Source: CAD feature listing. Evaluate the final solid. Frame: model axes, mm. Face numbers are marked on the shaded views. A direction names the side the tool comes from. Coordinates: 2 decimals unless noted, no trailing zeros. Loops run counter-clockwise (first coordinate to the right, second up) from the corner with the lowest first, then second, coordinate; pieces in that order, holes last. Notation, with made-up numbers: (28.5, -37) -> (76.5, -37) arc R5 ccw to (76.5, -29) -> close; hole circle Ø3 at (76, -2). An arc over 180 degrees is marked (long way). Answer as CSV lines item,"result".
from build123d import *

# Parameters (mm, degrees)
F1_DEPTH = 6.35
F3_DEPTH = 31.75
F5_DEPTH = 25.4
F6_R     = 2.5
F7_DEPTH = 25.4
F8_R     = 6.35


with BuildPart() as f1:
    # F0 (on Front) → F1 (new body)
    with BuildSketch(Plane.XZ):
        Polygon((0, 84.328), (0, 0), (26.416, 0), (33.3502, 46.99), (6.35, 71.628), (6.35, 84.328), align=None)
    extrude(amount=F1_DEPTH)

    # F2 (on face) → F3 (join)
    with BuildSketch(Plane.XZ.offset(6.35)):
        Polygon((0, 84.328), (0, 0), (6.35, 0), (6.35, 71.628), (6.35, 84.328), align=None)
    extrude(amount=F3_DEPTH)

    # F4 (on face) → F5 (cut)
    with BuildSketch(Plane.XZ.offset(6.35)):
        with BuildLine():
            Line((19.558, 12.9921), (14.478, 12.9921))
            ThreePointArc((14.478, 12.9921), (10.5029, 9.017), (14.478, 5.0419))
            Line((14.478, 5.0419), (19.558, 5.0419))
            ThreePointArc((19.558, 5.0419), (23.5331, 9.017), (19.558, 12.9921))
        make_face()
        with BuildLine():
            Line((24.1046, 45.9359), (19.0246, 45.9359))
            ThreePointArc((19.0246, 45.9359), (15.0495, 41.9608), (19.0246, 37.9857))
            Line((19.0246, 37.9857), (24.1046, 37.9857))
            ThreePointArc((24.1046, 37.9857), (28.0797, 41.9608), (24.1046, 45.9359))
        make_face()
    extrude(amount=-F5_DEPTH, mode=Mode.SUBTRACT)

    # F6 (on face) → F7 (cut)
    with BuildSketch(Plane.YZ.offset(6.35)):
        with Locations((-23.8125, 46.228)):
            Circle(F6_R)
        with Locations((-23.8125, 72.898)):
            Circle(F6_R)
    extrude(amount=-F7_DEPTH, mode=Mode.SUBTRACT)

    # F8
    f8_edges = [f1.edges().sort_by_distance(p)[0] for p in [
        (26.416, -3.175, 0),
        (33.3502, -3.175, 46.99),
        (6.35, -3.175, 71.628),
        (3.175, 0, 84.328),
        (3.175, -38.1, 84.328),
        (3.175, -38.1, 0),
    ]]
    fillet(f8_edges, radius=F8_R)


solid = f1.part
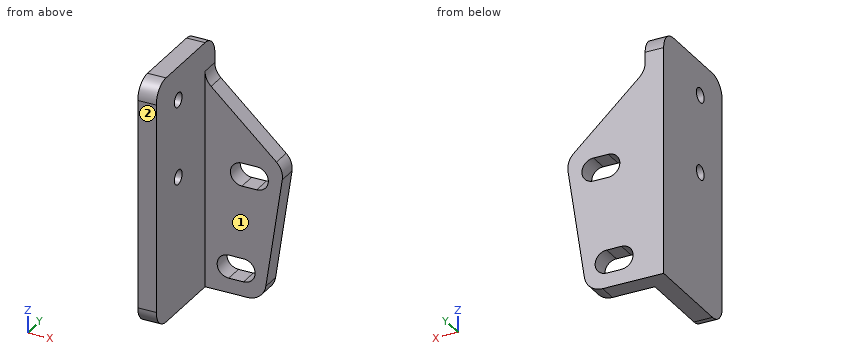
(1) Cut plane A-A (x = 22). Return the cut outline in (y, z).
Computed values:
outline,"(-6.35, 0.09) -> (0, 0.09) -> (0, 5.88) -> (-6.35, 5.88) -> close; (-6.35, 12.15) -> (0, 12.15) -> (0, 37.99) -> (-6.35, 37.99) -> close; (-6.35, 45.94) -> (0, 45.94) -> (0, 57.35) -> (-6.35, 57.35) -> close"
(2) Access query for the marked faces 1 and 2. Directions: +Z, -Z, +X, -X, +Y, -Y. A direction counts if a zero-diameter tool reaches every point of the face in a straight line with its end or side. Return the directions, or none.
Computed values:
face 1,"+Z, -Z, +X, -Y"
face 2,"+Z, -Z, +X, -X, -Y"
(3) Cut plane C-C (y = -22.5). Return the cut outline in (x, z).
Computed values:
outline,"(0, 0) -> (6.35, 0) -> (6.35, 44.1) -> (0, 44.1) -> close; (0, 48.36) -> (6.35, 48.36) -> (6.35, 70.77) -> (0, 70.77) -> close; (0, 75.03) -> (6.35, 75.03) -> (6.35, 84.33) -> (0, 84.33) -> close"
(4) Cut plane B-B (z = 11). Return the cut outline in (x, y), then the cut area to 3 significant figures.
Computed values:
outline,"(0, -38.1) -> (6.35, -38.1) -> (6.35, -6.35) -> (11.03, -6.35) -> (11.03, 0) -> (0, 0) -> close; (23, -6.35) -> (28.04, -6.35) -> (28.04, 0) -> (23, 0) -> close"
area,"304 mm^2"
(5) Material intervals for L1, parallel to Z at x = 19.5, y = -6; L2, parallel to X at y = -7.5, z = 23; L3, parallel to Y at x = 20, z = 52, sorted ascending. Write a range as [from, to].
Computed values:
L1,"[0, 5.04], [12.99, 37.99], [45.94, 59.63]"
L2,"[0, 6.35]"
L3,"[-6.35, 0]"
(6) Pin query (flat end, axial travel): pin 1 Ø8 at (y, z) = (-27.5, 33.5) entering from -X; pin 2 Ø5.5 at (x, y) = (17.5, -2.5) entering from +Z; pin 3 Ø11.5 at (y, z) = (-18.5, 48.5) entering from +X; pin 4 Ø13.5 at (x, z) = (24.5, 22.5) entering from -Y. Return the tip coordinate at first contact, or that it passes through.
Computed values:
pin 1,"x = 0"
pin 2,"z = 63.96"
pin 3,"x = 6.35"
pin 4,"y = -6.35"
(7) Cut plane D-D (x = 12.5). Return the cut outline in (y, z).
Computed values:
outline,"(-6.35, 0) -> (0, 0) -> (0, 5.57) -> (-6.35, 5.57) -> close; (-6.35, 12.47) -> (0, 12.47) -> (0, 66.02) -> (-6.35, 66.02) -> close"
